```python
from build123d import *

# Parameters (mm, degrees)
SKETCH_1_W        = 100
SKETCH_1_H        = 150
EXTRUDE_1_DEPTH   = 2
CHAMFER_1_SIZE    = 2
HOLE_WIZARD_M81_D = 9


with BuildPart() as part:
    # Эскиз1 → Бобышка-Вытянуть1 (new body)
    with BuildSketch(Plane.XY):
        Rectangle(SKETCH_1_W, SKETCH_1_H)
    extrude(amount=EXTRUDE_1_DEPTH)

    # Фаска1
    chamfer_1_edges = [part.edges().sort_by_distance(p)[0] for p in [
        (50, -75, 1),
        (-50, -75, 1),
        (-50, 75, 1),
        (50, 75, 1),
    ]]
    chamfer(chamfer_1_edges, length=CHAMFER_1_SIZE)

    # Отверстие с зазором M81 (through all)
    with Locations(Plane.XY.offset(2)):
        with Locations((-25, 50), (25, 50), (25, 0), (-25, 0), (-25, -50), (25, -50)):
            Hole(HOLE_WIZARD_M81_D / 2)


solid = part.part
```
Input: part model. Units: mm. Frame: model coordinates. Round coordinates to 2 decimals unless told otherwise and drop trailing zeros. Order: outer loops, then holes, each group sorted by start corner. A loop starts at its lowest first (then second) coordinate and runs counter-clockwise, first axis right, second up. Notation, with made-up numbers: (61.25, 72) - (119.25, 72) arc R26 cw to (119.25, 97) - close; hole circle Ø5 at (-14, 26.25). An arc over 180 degrees is marked (long way). Answer in a Markdown table with one row per item.
Item 1: Mould query, pull axis Y, two halves, no side actions, for faces 1 (the cylindrical face through (-24.02, -54.39, 0.99)), 2 (the flat face through (-1, 1, 0)). Classes: released by +Y, released by -Y, zero draft, split by the parting line, or undercut.
Model answer:
| item | result |
|---|---|
| face 1 | undercut |
| face 2 | zero draft |
Item 2: Line query: line 1 (Y direction, x = -25, z = 0.9); line 2 (X direction, y = 50.5, z = 1.5); line 3 (Y direction, x = 22, z = 1.6). Output: solid intervals per line, ascending.
Model answer:
| item | result |
|---|---|
| line 1 | y = -75 to -54.5, -45.5 to -4.5, 4.5 to 45.5, 54.5 to 75 |
| line 2 | x = -50 to -29.47, -20.53 to 20.53, 29.47 to 50 |
| line 3 | y = -75 to -53.35, -46.65 to -3.35, 3.35 to 46.65, 53.35 to 75 |
Item 3: Section query B-B (x = 25). Return the cut outline in (y, z), then the cut area to 3 significant figures.
Model answer:
| item | result |
|---|---|
| outline | (-75, 0) - (-54.5, 0) - (-54.5, 2) - (-75, 2) - close; (-45.5, 0) - (-4.5, 0) - (-4.5, 2) - (-45.5, 2) - close; (4.5, 0) - (45.5, 0) - (45.5, 2) - (4.5, 2) - close; (54.5, 0) - (75, 0) - (75, 2) - (54.5, 2) - close |
| area | 246 mm² |
Item 4: Section query A-A (y = 0). Return the cut outline in (x, z).
Model answer:
| item | result |
|---|---|
| outline | (-50, 0) - (-29.5, 0) - (-29.5, 2) - (-50, 2) - close; (-20.5, 0) - (20.5, 0) - (20.5, 2) - (-20.5, 2) - close; (29.5, 0) - (50, 0) - (50, 2) - (29.5, 2) - close |
Item 5: Section query D-D (y = 48). Return the cut outline in (x, z).
Model answer:
| item | result |
|---|---|
| outline | (-50, 0) - (-29.03, 0) - (-29.03, 2) - (-50, 2) - close; (-20.97, 0) - (20.97, 0) - (20.97, 2) - (-20.97, 2) - close; (29.03, 0) - (50, 0) - (50, 2) - (29.03, 2) - close |
Item 6: Section query C-C (z = 1.1). Return the cut outline in (x, y), then the cut area to 3 significant figures.
Model answer:
| item | result |
|---|---|
| outline | (-50, -73) - (-48, -75) - (48, -75) - (50, -73) - (50, 73) - (48, 75) - (-48, 75) - (-50, 73) - close; hole circle Ø9 at (-25, -50); hole circle Ø9 at (-25, 0); hole circle Ø9 at (-25, 50); hole circle Ø9 at (25, -50); hole circle Ø9 at (25, 0); hole circle Ø9 at (25, 50) |
| area | 14,600 mm² |
Item 7: Pin query (flat end, axial travel): pin 1 (5.5 mm diameter, centred on x = 25, y = 50, fed in from +Z). Return the tip coordinate at first contact, or that it passes through.
Model answer:
| item | result |
|---|---|
| pin 1 | passes through |
